from build123d import *

# Parameters (mm, degrees)
F0_R     = 11.05
F0_R_2   = 6.55
F1_DEPTH = 7
F2_R     = 5
F3_SIZE  = 2.5
F4_R     = 6.55
F4_R_2   = 6.15
F5_DEPTH = 5
F6_SIZE  = 0.7
F8_DEPTH = 25


with BuildPart() as f1:
    # F0 (on Top) → F1 (new body)
    with BuildSketch(Plane.XY):
        with BuildLine():
            Line((8.6602540378, 5), (14.0883655764, 19.8504412435))
            ThreePointArc((14.0883655764, 19.8504412435), (0, 40), (-14.0883655764, 19.8504412435))
            Line((-14.0883655764, 19.8504412435), (-8.6602540378, 5))
            Line((-8.6602540378, 5), (-24.2351691813, 2.2756618652))
            ThreePointArc((-24.2351691813, 2.2756618652), (-34.6410161514, -20), (-10.146803605, -22.1261031087))
            Line((-10.146803605, -22.1261031087), (0, -10))
            Line((0, -10), (10.146803605, -22.1261031087))
            ThreePointArc((10.146803605, -22.1261031087), (34.6410161514, -20), (24.2351691813, 2.2756618652))
            Line((24.2351691813, 2.2756618652), (8.6602540378, 5))
        make_face()
        with Locations((-21.6506350946, -12.5)):
            Circle(F0_R, mode=Mode.SUBTRACT)
        with Locations((21.6506350946, -12.5)):
            Circle(F0_R, mode=Mode.SUBTRACT)
        Circle(F0_R_2, mode=Mode.SUBTRACT)
        with Locations((0, 25)):
            Circle(F0_R, mode=Mode.SUBTRACT)
    extrude(amount=F1_DEPTH)

    # F2
    f2_edges = [f1.edges().sort_by_distance(p)[0] for p in [
        (0, -10, 3.5),
        (8.660254, 5, 3.5),
        (-8.660254, 5, 3.5),
    ]]
    fillet(f2_edges, radius=F2_R)

    # F3
    f3_edges = [f1.edges().sort_by_distance(p)[0] for p in [
        (-19.390694, 3.123049, 7),
        (-6.990707, -18.354358, 0),
        (12.399987, 15.231309, 0),
        (12.399987, 15.231309, 7),
        (11.077604, 6.395657, 0),
        (0, 40, 0),
        (19.390694, 3.123049, 0),
        (-12.399987, 15.231309, 0),
        (34.641016, -20, 0),
        (-11.077604, 6.395657, 0),
        (6.990707, -18.354358, 0),
        (-19.390694, 3.123049, 0),
        (0, -12.791315, 0),
        (-34.641016, -20, 0),
        (11.077604, 6.395657, 7),
        (0, 40, 7),
        (19.390694, 3.123049, 7),
        (-12.399987, 15.231309, 7),
        (34.641016, -20, 7),
        (-11.077604, 6.395657, 7),
        (6.990707, -18.354358, 7),
        (0, -12.791315, 7),
        (-34.641016, -20, 7),
        (-6.990707, -18.354358, 7),
    ]]
    chamfer(f3_edges, length=F3_SIZE)

    # F4 (on face) → F5 (join)
    with BuildSketch(Plane(origin=(0, 0, 0), x_dir=(1, 0, 0), z_dir=(0, 0, -1))):
        Circle(F4_R)
        Circle(F4_R_2, mode=Mode.SUBTRACT)
    extrude(amount=-F5_DEPTH)

    # F6
    f6_edges = [f1.edges().sort_by_distance(p)[0] for p in [
        (-6.55, 0, 7),
        (-32.700635, -12.5, 7),
        (10.600635, -12.5, 7),
        (-11.05, 25, 7),
        (-32.700635, -12.5, 0),
        (10.600635, -12.5, 0),
        (-11.05, 25, 0),
    ]]
    chamfer(f6_edges, length=F6_SIZE)

    # F7 (on face) → F8 (cut)
    with BuildSketch(Plane.XY.offset(7)):
        with BuildLine():
            ThreePointArc((-4.1925255318, -8.5805145338), (-8.2705426061, -4.775), (-9.5272063297, 0.6594236504))
            ThreePointArc((-9.5272063297, 0.6594236504), (-11.4782376336, -0.3808245165), (-13.6062935442, -0.9808390488))
            ThreePointArc((-13.6062935442, -0.9808390488), (-9.4829781714, -5.475), (-7.6525783054, -11.2929763362))
            ThreePointArc((-7.6525783054, -11.2929763362), (-6.0689225225, -9.7500331232), (-4.1925255318, -8.5805145338))
        make_face()
        with BuildLine():
            ThreePointArc((-5.3346807979, 7.9210908835), (0, 9.55), (5.3346807979, 7.9210908835))
            ThreePointArc((5.3346807979, 7.9210908835), (5.4093151112, 10.1308576396), (5.9537152388, 12.273815385))
            ThreePointArc((5.9537152388, 12.273815385), (0, 10.95), (-5.9537152388, 12.273815385))
            ThreePointArc((-5.9537152388, 12.273815385), (-5.4093151112, 10.1308576396), (-5.3346807979, 7.9210908835))
        make_face()
        with BuildLine():
            ThreePointArc((9.5272063297, 0.6594236504), (8.2705426061, -4.775), (4.1925255318, -8.5805145338))
            ThreePointArc((4.1925255318, -8.5805145338), (6.0689225225, -9.7500331232), (7.6525783054, -11.2929763362))
            ThreePointArc((7.6525783054, -11.2929763362), (9.4829781714, -5.475), (13.6062935442, -0.9808390488))
            ThreePointArc((13.6062935442, -0.9808390488), (11.4782376336, -0.3808245165), (9.5272063297, 0.6594236504))
        make_face()
    extrude(amount=-F8_DEPTH, mode=Mode.SUBTRACT)


solid = f1.part
The listing builds one solid part. Answer for the finished solid, in the listing's coordinates (mm). A direction names the side the tool comes from. Coordinates: 2 decimals unless noted, no trailing zeros. Order: outer loops, then holes, each group sorted by start corner. A loop starts at its lowest first (then second) coordinate and runs counter-clockwise, first axis right, second up.
Q1. A cutting plane is placed at C-C, the plane z = 3.5. Write down the section's boundary in (x, y).
Q2. Given P1, Ø8, axis at x = -14.5, y = 6.5, coming from the -Z side; P2, Ø3, axis at y = -14.5, z = 5, coming from the -X side, each flat-ended and moving along its own axis, determine where each tip first touches the part or whether it passes through.
Q3. For a pull along Y with two mould halves and no side action, classify faces 1 (the face through (-30.42, -19.22, 3.46)), 2 (the face through (-32.78, -18.53, 0.16)), 3 (the face through (7.89, -17.51, 1.27)) as pulls with the +Y half, pulls with the -Y half, needs draft (parallel to the pull), parting line crosses it, or undercut.
Q4. A cutting plane is placed at A-A, the plane x = 0. State how many separate pieces and enclosed holes the cut face has, and give its area (3 significant figures).
Q5. Consider line 1 (Y direction, x = 0, z = 3.6); line 2 (X direction, y = 0, z = 5.3); line 3 (X direction, y = -16.5, z = 1.5). Determine where each line is inside the solid, lowest interval first.
Q6. Which of the six approach directions +Z, -Z, +X, -X, +Y, -Y give full straight-line access (tool end or side, diameter ignored) to faces 4 (the face through (6.947, -18.302, 3.486)), 5 (the face through (-7.98, -17.62, 1.27)), 6 (the face through (-0.853, 6.494, 5.641))?
Q7. A cutting plane is placed at B-B, the plane y = 25. Write down the section's boundary in (x, z), and give its area (3 significant figures).
Answers follow:
1. outline: (-24.24, 2.28) arc R15 ccw (long way) to (-10.15, -22.13) - (-3.83, -14.58) arc R5 cw to (3.83, -14.58) - (10.15, -22.13) arc R15 ccw (long way) to (24.24, 2.28) - (14.55, 3.97) arc R5 cw to (10.71, 10.61) - (14.09, 19.85) arc R15 ccw (long way) to (-14.09, 19.85) - (-10.71, 10.61) arc R5 cw to (-14.55, 3.97) - close; hole circle Ø22.1 at (-21.65, -12.5); hole (-13.61, -0.98) arc R14.05 cw to (-7.65, -11.29) arc R10.3 cw to (-4.19, -8.58) arc R9.55 cw to (-9.53, 0.66) arc R10.3 cw to start; hole circle Ø22.1 at (0, 25); hole circle Ø12.3 at (0, 0); hole (-5.95, 12.27) arc R10.3 cw to (-5.33, 7.92) arc R9.55 cw to (5.33, 7.92) arc R10.3 cw to (5.95, 12.27) arc R14.05 cw to start; hole (4.19, -8.58) arc R10.3 cw to (7.65, -11.29) arc R14.05 cw to (13.61, -0.98) arc R10.3 cw to (9.53, 0.66) arc R9.55 cw to start; hole circle Ø22.1 at (21.65, -12.5)
2. P1: stops at z = 0.94
2. P2: stops at x = -36.64
3. face 1: undercut
3. face 2: parting line crosses it
3. face 3: pulls with the -Y half
4. separate pieces: 4
4. enclosed holes: 0
4. area: 103 mm2
5. line 1: y = -12.79 to -6.15, 6.15 to 9.55, 10.95 to 13.95, 36.05 to 40
5. line 2: x = -28.39 to -10.64, -9.55 to -6.55, 6.55 to 9.55, 10.64 to 28.39
5. line 3: x = -35.07 to -31.95, -11.35 to -6.74, 6.74 to 11.35, 31.95 to 35.07
6. face 4: +Z, -Z, -Y
6. face 5: -Z, -Y
6. face 6: +Z
7. outline: (-15, 2.5) - (-12.5, 0) - (-11.75, 0) - (-11.05, 0.7) - (-11.05, 6.3) - (-11.75, 7) - (-12.5, 7) - (-15, 4.5) - close; (11.05, 0.7) - (11.75, 0) - (12.5, 0) - (15, 2.5) - (15, 4.5) - (12.5, 7) - (11.75, 7) - (11.05, 6.3) - close
7. area: 41.8 mm2
